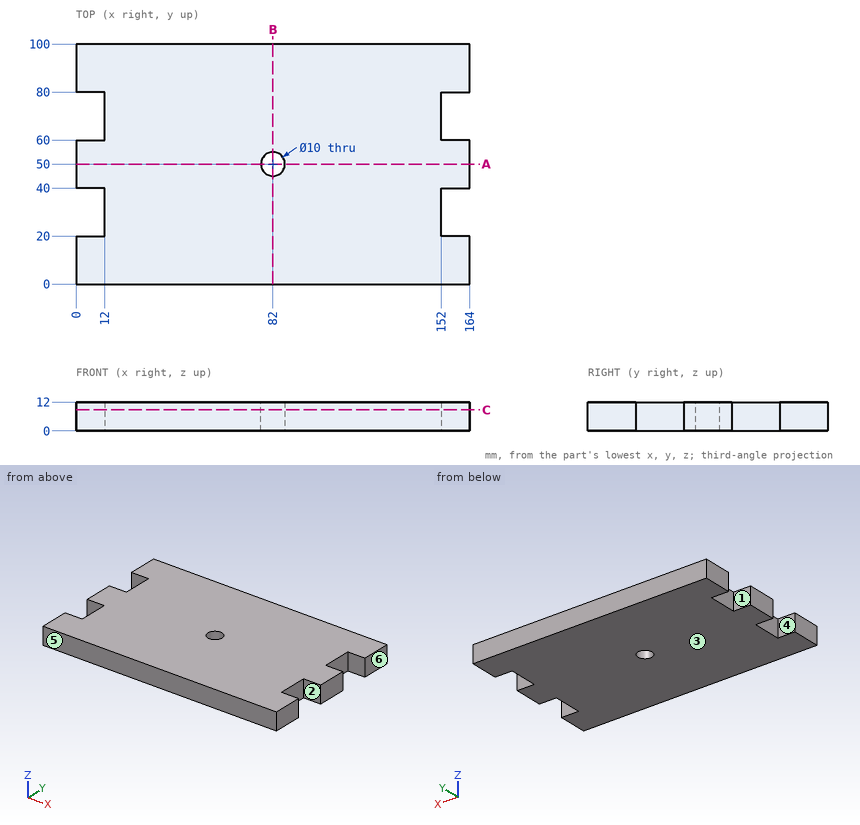
Study the drawing (mm; zero at the part's minimum x, y, z) and answer. A direction names the side the tool comes from. Coordinates: 2 decimals unless noted, no trailing zeros. Order: outer loops, then holes, each group sorted by start corner. A loop starts at its lowest first (then second) coordinate and runs counter-clockwise, first axis right, second up. Notation, with made-up numbers: (-36.5, -16.5) -> (-13.5, -16.5) arc R21 ccw to (-13.5, 15.5) -> close; hole circle Ø4 at (77, 84.25). An arc over 180 degrees is marked (long way). Answer in a Markdown table with one row per item. Add a question column.
Item 1: Find the intervals of material crossed by L1, parallel to Y at x = 82, z = 8.5; L2, parallel to Y at x = 157, z = 5.5; L3, parallel to X at y = 37, z = 2.75, in increasing order. Write a range as from..to.
Item 2: Determine the mould class of the marked faces 4, 5 and 6 for opening direction Y: +Y half, -Y half, draft (parallel to the pull), parting line (faces both ways), or undercut.
Item 3: Find section B-B (x = 82). Write down the section's boundary in (y, z).
Item 4: Each of these flat-tipped pins is pushed along its axis until it touches: P1, Ø6, axis at x = 82, y = 50, coming from the -Z side; P2, Ø3.5, axis at y = 27.5, z = 6, coming from the -X side; P3, Ø6, axis at y = 67.5, z = 4, coming from the +X side. Where does it stop, or does it pass through?
Item 5: Find section C-C (z = 8.75). Write down the section's boundary in (x, y), then the cut area to 3 significant figures.
Item 6: Which of the six approach directions +Z, -Z, +X, -X, +Y, -Y give full straight-line access (tool end or side, diameter ignored) to the marked faces 1, 2 and 3?
Item 7: Find section A-A (y = 50). Write down the section's boundary in (x, z), then the cut area to 3 significant figures.
Result set:
| question | item | result |
|---|---|---|
| 1 | L1 | y = 0..45, 55..100 |
| 1 | L2 | y = 0..20, 40..60, 80..100 |
| 1 | L3 | x = 12..152 |
| 2 | face 4 | undercut |
| 2 | face 5 | -Y half |
| 2 | face 6 | draft |
| 3 | outline | (0, 0) -> (45, 0) -> (45, 12) -> (0, 12) -> close; (55, 0) -> (100, 0) -> (100, 12) -> (55, 12) -> close |
| 4 | P1 | passes through |
| 4 | P2 | stops at x = 12 |
| 4 | P3 | stops at x = 152 |
| 5 | outline | (0, 0) -> (164, 0) -> (164, 20) -> (152, 20) -> (152, 40) -> (164, 40) -> (164, 60) -> (152, 60) -> (152, 80) -> (164, 80) -> (164, 100) -> (0, 100) -> (0, 80) -> (12, 80) -> (12, 60) -> (0, 60) -> (0, 40) -> (12, 40) -> (12, 20) -> (0, 20) -> close; hole circle Ø10 at (82, 50) |
| 5 | area | 15,400 mm² |
| 6 | face 1 | +Z, -Z, -X |
| 6 | face 2 | +Z, -Z, +X |
| 6 | face 3 | -Z, +X, -X, +Y, -Y |
| 7 | outline | (0, 0) -> (77, 0) -> (77, 12) -> (0, 12) -> close; (87, 0) -> (164, 0) -> (164, 12) -> (87, 12) -> close |
| 7 | area | 1,850 mm² |
